Geometry check sheet. Reference: the model listing, model coordinates, mm. A direction names the side the tool comes from. Round coordinates to 2 decimals unless told otherwise and drop trailing zeros. Order: outer loops, then holes, each group sorted by start corner. A loop starts at its lowest first (then second) coordinate and runs counter-clockwise, first axis right, second up. Notation, with made-up numbers: (47.25, 44.5) - (61.25, 44.5) arc R15 ccw to (61.25, 53.5) - close; hole circle Ø6 at (52.5, 88.5). An arc over 180 degrees is marked (long way). Answer as CSV lines item,"result". Start each with the question number.
```python
from build123d import *

# Parameters (mm, degrees)
SKETCH_1_R          = 200
SKETCH_1_R_2        = 193.5
EXTRUDE_1_DEPTH     = 39
SKETCH_1_5_R        = 193.5
SKETCH_1_5_R_2      = 189.6
EXTRUDE_2_DEPTH     = 9.8
CUT_EXTRUDE_START   = -23.1
CUT_EXTRUDE_1_DEPTH = 23.1


with BuildPart() as part:
    # 草图1 → 凸台-拉伸1 (new body)
    with BuildSketch(Plane(origin=(0, 0, 0), x_dir=(1, 0, 0), z_dir=(0, 1, 0))):
        with Locations(Location((0, 0, 0), (0, 0, 270))):
            Circle(SKETCH_1_R)
        with Locations(Location((0, 0, 0), (0, 0, 270))):
            Circle(SKETCH_1_R_2, mode=Mode.SUBTRACT)
    extrude(amount=EXTRUDE_1_DEPTH)

    # 草图1<5> → 凸台-拉伸2 (add)
    with BuildSketch(Plane(origin=(0, 0, 0), x_dir=(1, 0, 0), z_dir=(0, 1, 0))):
        with Locations(Location((0, 0, 0), (0, 0, 270))):
            Circle(SKETCH_1_5_R)
        with Locations(Location((0, 0, 0), (0, 0, 270))):
            Circle(SKETCH_1_5_R_2, mode=Mode.SUBTRACT)
    extrude(amount=EXTRUDE_2_DEPTH)

    # 草图4 → 切除-拉伸1 (cut)
    with BuildSketch(Plane(origin=(0, 39, 0), x_dir=(1, 0, 0), z_dir=(0, 1, 0)).offset(CUT_EXTRUDE_START)):
        with BuildLine():
            Line((-50.081485227, -186.906647387), (-51.763809021, -193.185165258))
            ThreePointArc((-51.763809021, -193.185165258), (0, -200), (51.763809021, -193.185165258))
            Line((51.763809021, -193.185165258), (50.081485227, -186.906647387))
            ThreePointArc((50.081485227, -186.906647387), (0, -193.5), (-50.081485227, -186.906647387))
        make_face()
    extrude(amount=CUT_EXTRUDE_1_DEPTH, mode=Mode.SUBTRACT)


solid = part.part
```
1. Access from +Z, -Z, +X, -X, +Y, -Y to the whole of each face (thin tool, end or side, straight path). Record for faces 1 (the face through (-76.6, 19.23, 184.75)), 2 (the face through (-1, 15.9, 195)), 3 (the face through (-128, 9.8, 142)).
2. Section check B-B on z = -96. Record the boundary of the cut face in (x, y), plus the area to 3 significant figures.
3. Section check A-A on x = 0. Record the boundary of the cut face in (y, z), plus the area to 3 significant figures.
4. Thickness scan on probe 1 along X at (y, z) = (18.25, 0); probe 2 along X at (y, z) = (3, 0); probe 3 along Z at (x, y) = (124, 7.5). Record the ranges inside material, lowest first.
5. Go/stop test with flat-tipped pins: pin 1 Ø5 at (y, z) = (10, 51.5) entering from -X; pin 2 Ø4 at (x, y) = (80, 16) entering from -Z; pin 3 Ø10.5 at (x, z) = (13.5, 191) entering from +Y. Record where each tip stops, or that it passes through.
6. Section check C-C on y = 20.5. Record the boundary of the cut face in (x, z).
Numbers:
1,face 1,"+Y, -Y"
1,face 2,"+Z, +Y"
1,face 3,"+Y"
2,outline,"(-175.45, 0) - (-163.5, 0) - (-163.5, 9.8) - (-168.01, 9.8) - (-168.01, 39) - (-175.45, 39) - close; (163.5, 0) - (175.45, 0) - (175.45, 39) - (168.01, 39) - (168.01, 9.8) - (163.5, 9.8) - close"
2,area,"669 mm2"
3,outline,"(0, -200) - (39, -200) - (39, -193.5) - (9.8, -193.5) - (9.8, -189.6) - (0, -189.6) - close; (0, 189.6) - (9.8, 189.6) - (9.8, 193.5) - (15.9, 193.5) - (15.9, 200) - (0, 200) - close"
3,area,"433 mm2"
4,probe 1,"x = -200 to -193.5, 193.5 to 200"
4,probe 2,"x = -200 to -189.6, 189.6 to 200"
4,probe 3,"z = -156.92 to -143.43, 143.43 to 156.92"
5,pin 1,"stops at x = -193.9"
5,pin 2,"stops at z = -184.16"
5,pin 3,"stops at y = 15.9"
6,outline,"(-51.76, 193.19) arc R200 ccw (long way) to (51.76, 193.19) - (50.08, 186.91) arc R193.5 cw (long way) to (-50.08, 186.91) - close"
